CAD build for the part. Positions are in the model's coordinates, mm. A direction names the side the tool comes from. Coordinates: 2 decimals unless noted, no trailing zeros. Loops run counter-clockwise (first coordinate to the right, second up) from the corner with the lowest first, then second, coordinate; pieces in that order, holes last. Notation, with made-up numbers: (-20, -5.5) -> (20, -5.5) arc R11 cw to (20, 0.5) -> close; hole circle Ø5 at (-25, 80). An arc over 180 degrees is marked (long way). Write item = value, one per line. Start each with the question number.
(1) Flat gauge pins, fed straight in: P1, Ø1, axis at x = 4.5, z = 5.5, coming from the -Y side; P2, Ø1.5, axis at x = 2.5, z = 14.5, coming from the -Y side; P3, Ø5, axis at x = 3.5, z = 8.5, coming from the -Y side. Where does each tip first touch, or does it go through?
(2) Band-saw the part on A-A (x = 0). Write the cut outline in (y, z), and give its area (3 significant figures).
(3) Drill centre lines: line 1 (X direction, y = -3, z = 15); line 2 (Y direction, x = -4.75, z = 4); line 3 (X direction, y = 0.75, z = -20). Where is each one in solid material? Low to high. Write a range as from..to.
(4) Tool access for faces 1 (the face through (-3, 3, -14)), 2 (the face through (0, 0, -27)): list every direction of +Z, -Z, +X, -X, +Y, -Y with a clear straight run to the whole face (end or side of a thin tool).
(5) Band-saw the part on C-C (z = -12.5). Write the cut outline in (x, y).
```python
from build123d import *

# Parameters (mm, degrees)
CROQUIS1_R              = 6
SALIENTE_EXTRUIR1_DEPTH = 10
CROQUIS2_R              = 6
SALIENTE_EXTRUIR2_DEPTH = 10
CHAFL_N1_SIZE           = 10
CHAFL_N1_SIZE2          = 1.763269807
REDONDEO1_R             = 2
CROQUIS3_R              = 4.5
SALIENTE_EXTRUIR3_DEPTH = 14
CROQUIS4_R              = 4
SALIENTE_EXTRUIR4_DEPTH = 13
CHAFL_N2_SIZE           = 1
CHAFL_N2_SIZE2          = 0.176326981


with BuildPart() as part:
    # Croquis1 → Saliente-Extruir1 (new body)
    with BuildSketch(Plane.XY):
        Circle(CROQUIS1_R)
    extrude(amount=SALIENTE_EXTRUIR1_DEPTH)

    # Croquis2 → Saliente-Extruir2 (add)
    with BuildSketch(Plane.XY.offset(10)):
        Circle(CROQUIS2_R)
    extrude(amount=SALIENTE_EXTRUIR2_DEPTH)

    # Chaflán1
    chafl_n1_edges = [part.edges().sort_by_distance(p)[0] for p in [
        (-6, 0, 20),
    ]]
    chafl_n1_side = [part.faces().sort_by_distance(p)[0] for p in [
        (-6, 0, 10),
    ]]
    chamfer(chafl_n1_edges, length=CHAFL_N1_SIZE, length2=CHAFL_N1_SIZE2, reference=chafl_n1_side[0])

    # Redondeo1
    redondeo1_edges = [part.edges().sort_by_distance(p)[0] for p in [
        (-4.236730193, 0, 20),
    ]]
    fillet(redondeo1_edges, radius=REDONDEO1_R)

    # Croquis3 → Saliente-Extruir3 (add)
    with BuildSketch(Plane(origin=(0, 0, 0), x_dir=(-1, 0, 0), z_dir=(0, 0, -1))):
        with Locations(Location((0, 0, 0), (0, 0, 180))):
            Circle(CROQUIS3_R)
    extrude(amount=SALIENTE_EXTRUIR3_DEPTH)

    # Croquis4 → Saliente-Extruir4 (add)
    with BuildSketch(Plane(origin=(0, 0, -14), x_dir=(-1, 0, 0), z_dir=(0, 0, -1))):
        with Locations(Location((0, 0, 0), (0, 0, 180))):
            Circle(CROQUIS4_R)
    extrude(amount=SALIENTE_EXTRUIR4_DEPTH)

    # Chaflán2
    chafl_n2_edges = [part.edges().sort_by_distance(p)[0] for p in [
        (-4, 0, -27),
    ]]
    chafl_n2_side = [part.faces().sort_by_distance(p)[0] for p in [
        (-4, 0, -20.5),
    ]]
    chamfer(chafl_n2_edges, length=CHAFL_N2_SIZE, length2=CHAFL_N2_SIZE2, reference=chafl_n2_side[0])


solid = part.part
```
Findings below:
q1.P1 = -4.47
q1.P2 = -4.94
q1.P3 = -5.92
q2.outline = (-6, 0) -> (-4.5, 0) -> (-4.5, -14) -> (-4, -14) -> (-4, -26) -> (-3.82, -27) -> (3.82, -27) -> (4, -26) -> (4, -14) -> (4.5, -14) -> (4.5, 0) -> (6, 0) -> (6, 10) -> (4.53, 18.35) arc R2 ccw to (2.56, 20) -> (-2.56, 20) arc R2 ccw to (-4.53, 18.35) -> (-6, 10) -> close
q2.area = 451 mm²
q3.line_1 = -4.15..4.15
q3.line_2 = -3.67..3.67
q3.line_3 = -3.93..3.93
q4.face_1 = -Z
q4.face_2 = -Z, +X, -X, +Y, -Y
q5.outline = circle Ø9 at (0, 0)
